Geometry check sheet. Reference: the model listing, model coordinates, mm. A direction names the side the tool comes from. Coordinates: 2 decimals unless noted, no trailing zeros. Use CSV: the item, a comma, the result in double quotes. Start each with the question number.
1) Tool access check on faces 4 (the flat face through (-1, 2, 100)), 5 (the flat face through (91.4, 2.5, -73.6)). Record the directions out of +Z, -Z, +X, -X, +Y, -Y that give a thin tool (end or side, any length) a straight path to the whole face; none if there is none.
2) Thickness scan on probe 1 along Z at (x, y) = (90, 2); probe 2 along X at (y, z) = (3.6, -75); probe 3 along Z at (x, y) = (75, 3.35). Record the ranges inside material, lowest first. Write a range as [from, to].
3) Draft check along Z on faces 1 (the cylindrical face through (72.421, 3.732, -88.022)), 2 (the flat face through (-1, 2, -100)), 3 (the flat face through (-1, 0, -1)). Enter one of: released by +Z, released by -Z, zero draft, split by the parting line, or undercut.
4) Depth check by flat-ended pin: P1, Ø6, axis at x = 75, z = -90, coming from the +Y side. Enter the tip coordinate at first touch or a pass-through.
from build123d import *

# Parameters (mm, degrees)
SKETCH1_W                                     = 200
SKETCH1_H                                     = 200
BASE_PLATE_DEPTH                              = 5
CBORE_START                                   = 2.5
CBORE_FOR_M3_HEX_SOCKET_HEAD_CAP_SCR_2_R      = 3.25
CBORE_FOR_M3_HEX_SOCKET_HEAD_CAP_SCREW1_DEPTH = 2.5
CBORE_FOR_M3_HEX_SOCKET_HEAD_CAP_SCR_3_O_R    = 1.7
CBORE_FOR_M3_HEX_SOCKET_HEAD_CAP_SCR_3_DEPTH  = 2.5


# Read off the part's stored shape, not the designer's step: CBORE for M3 Hex Socket Head Cap Screw1
with BuildPart() as part:
    # Sketch1 → base_plate (new body)
    with BuildSketch(Plane(origin=(0, 0, 0), x_dir=(1, 0, 0), z_dir=(0, 1, 0))):
        Rectangle(SKETCH1_W, SKETCH1_H)
    extrude(amount=BASE_PLATE_DEPTH)

    # CBORE for M3 Hex Socket Head Cap Scr 2 → CBORE for M3 Hex Socket Head Cap Screw1 (cut)
    with BuildSketch(Plane(origin=(0, 0, 0), x_dir=(1, 0, 0), z_dir=(0, 1, 0)).offset(CBORE_START)):
        with Locations((90, 75)):
            Circle(CBORE_FOR_M3_HEX_SOCKET_HEAD_CAP_SCR_2_R)
        with Locations((75, 90)):
            Circle(CBORE_FOR_M3_HEX_SOCKET_HEAD_CAP_SCR_2_R)
    extrude(amount=CBORE_FOR_M3_HEX_SOCKET_HEAD_CAP_SCREW1_DEPTH, mode=Mode.SUBTRACT)

    # CBORE for M3 Hex Socket Head Cap Scr 3 o → CBORE for M3 Hex Socket Head Cap Scr 3 (cut)
    with BuildSketch(Plane(origin=(0, 0, 0), x_dir=(1, 0, 0), z_dir=(0, 1, 0))):
        with Locations((90, 75)):
            Circle(CBORE_FOR_M3_HEX_SOCKET_HEAD_CAP_SCR_3_O_R)
        with Locations((75, 90)):
            Circle(CBORE_FOR_M3_HEX_SOCKET_HEAD_CAP_SCR_3_O_R)
    extrude(amount=CBORE_FOR_M3_HEX_SOCKET_HEAD_CAP_SCR_3_DEPTH, mode=Mode.SUBTRACT)


solid = part.part
Evaluation:
1,face 4,"+Z, +X, -X, +Y, -Y"
1,face 5,"+Y"
2,probe 1,"[-100, -76.7], [-73.3, 100]"
2,probe 2,"[-100, 86.75], [93.25, 100]"
2,probe 3,"[-100, -93.25], [-86.75, 100]"
3,face 1,"undercut"
3,face 2,"released by -Z"
3,face 3,"zero draft"
4,P1,"y = 2.5"
